from build123d import *

# Parameters (mm, degrees)
SKETCH1_R                   = 1.5
BOSS_EXTRUDE3_DEPTH         = 20
M10X1_0_TAPPED_HOLE2_REACH  = 97.384
M10X1_0_TAPPED_HOLE2_BORE_R = 4.5
M10X1_0_TAPPED_HOLE3_REACH  = 97.384
M10X1_0_TAPPED_HOLE3_BORE_R = 4.5
M10X1_0_TAPPED_HOLE4_REACH  = 97.514
M10X1_0_TAPPED_HOLE4_BORE_R = 4.5
M10X1_0_TAPPED_HOLE5_REACH  = 97.514
M10X1_0_TAPPED_HOLE5_BORE_R = 4.5


with BuildPart() as part:
    # Sketch1 → Boss-Extrude3 (new body)
    with BuildSketch(Plane(origin=(0, 0, 0), x_dir=(1, 0, 0), z_dir=(0, 1, 0))):
        with BuildLine():
            Line((-44.503051854, 39.975242963), (-45, 40))
            ThreePointArc((-45, 40), (-48.535533906, 38.535533906), (-50, 35))
            Line((-50, 35), (-49.953621428, 34.32056292))
            Line((-49.953621428, 34.32056292), (-47.610889869, 0))
            Line((-47.610889869, 0), (-49.953621428, -34.32056292))
            Line((-49.953621428, -34.32056292), (-50, -35))
            ThreePointArc((-50, -35), (-48.535533906, -38.535533906), (-45, -40))
            Line((-45, -40), (0, -37.473505635))
            Line((0, -37.473505635), (45, -40))
            ThreePointArc((45, -40), (48.535533906, -38.535533906), (50, -35))
            Line((50, -35), (49.982372149, -34.580514872))
            Line((49.982372149, -34.580514872), (48.529209365, 0))
            Line((48.529209365, 0), (49.982372149, 34.580514872))
            Line((49.982372149, 34.580514872), (50, 35))
            ThreePointArc((50, 35), (48.535533906, 38.535533906), (45, 40))
            Line((45, 40), (44.503051854, 39.975242963))
            Line((44.503051854, 39.975242963), (0, 37.758183271))
            Line((0, 37.758183271), (-44.503051854, 39.975242963))
        make_face()
        with Locations(Location((-45, -35, 0), (0, 0, 270))):
            Circle(SKETCH1_R, mode=Mode.SUBTRACT)
        with Locations(Location((45, -35, 0), (0, 0, 270))):
            Circle(SKETCH1_R, mode=Mode.SUBTRACT)
        with Locations(Location((-45, 35, 0), (0, 0, 270))):
            Circle(SKETCH1_R, mode=Mode.SUBTRACT)
        with BuildLine():
            Line((40.685277967, -32.473505635), (-40.685277967, -32.473505635))
            ThreePointArc((-40.685277967, -32.473505635), (-41.520684905, -31.409127338), (-42.610889869, -30.607716678))
            Line((-42.610889869, -30.607716678), (-42.610889869, 30.607716678))
            ThreePointArc((-42.610889869, 30.607716678), (-41.406196107, 31.523712673), (-40.530743043, 32.758183271))
            Line((-40.530743043, 32.758183271), (40.530743043, 32.758183271))
            ThreePointArc((40.530743043, 32.758183271), (41.770434724, 31.182945097), (43.529209365, 30.221216169))
            Line((43.529209365, 30.221216169), (43.529209365, -30.221216169))
            ThreePointArc((43.529209365, -30.221216169), (41.895770439, -31.080336898), (40.685277967, -32.473505635))
        make_face(mode=Mode.SUBTRACT)
        with Locations(Location((45, 35, 0), (0, 0, 270))):
            Circle(SKETCH1_R, mode=Mode.SUBTRACT)
    extrude(amount=BOSS_EXTRUDE3_DEPTH)

    # M10x1.0 Tapped Hole2 bore → M10x1.0 Tapped Hole2 (cut, up to next)
    with BuildSketch(Plane(origin=(2.097313344, 0, 37.355753405), x_dir=(0.9984276240489233, 0, -0.05605603924665131), z_dir=(0.05605603924665131, 0, 0.9984276240489233)), mode=Mode.PRIVATE) as m10x1_0_tapped_hole2_sk1:
        with Locations((-24.636050477, 10)):
            Circle(M10X1_0_TAPPED_HOLE2_BORE_R)
    m10x1_0_tapped_hole2_tool1 = extrude(m10x1_0_tapped_hole2_sk1.sketch, amount=-M10X1_0_TAPPED_HOLE2_REACH, mode=Mode.PRIVATE) & part.part
    add(m10x1_0_tapped_hole2_tool1.solids().sort_by_distance((-22.5, 10, 38.736753))[0], mode=Mode.SUBTRACT)

    # M10x1.0 Tapped Hole3 bore → M10x1.0 Tapped Hole3 (cut, up to next)
    with BuildSketch(Plane(origin=(-2.097313344, 0, 37.355753405), x_dir=(0.9984276240489233, 0, 0.056056039246651354), z_dir=(-0.056056039246651354, 0, 0.9984276240489233)), mode=Mode.PRIVATE) as m10x1_0_tapped_hole3_sk1:
        with Locations((24.636050477, 10)):
            Circle(M10X1_0_TAPPED_HOLE3_BORE_R)
    m10x1_0_tapped_hole3_tool1 = extrude(m10x1_0_tapped_hole3_sk1.sketch, amount=-M10X1_0_TAPPED_HOLE3_REACH, mode=Mode.PRIVATE) & part.part
    add(m10x1_0_tapped_hole3_tool1.solids().sort_by_distance((22.5, 10, 38.736753))[0], mode=Mode.SUBTRACT)

    # M10x1.0 Tapped Hole4 bore → M10x1.0 Tapped Hole4 (cut, up to next)
    with BuildSketch(Plane(origin=(-1.876385916, 0, -37.664705196), x_dir=(-0.9987613810598752, 0, 0.049756443837666), z_dir=(-0.049756443837666, 0, -0.9987613810598752)), mode=Mode.PRIVATE) as m10x1_0_tapped_hole4_sk1:
        with Locations((-24.406616413, 10)):
            Circle(M10X1_0_TAPPED_HOLE4_BORE_R)
    m10x1_0_tapped_hole4_tool1 = extrude(m10x1_0_tapped_hole4_sk1.sketch, amount=-M10X1_0_TAPPED_HOLE4_REACH, mode=Mode.PRIVATE) & part.part
    add(m10x1_0_tapped_hole4_tool1.solids().sort_by_distance((22.5, 10, -38.879092))[0], mode=Mode.SUBTRACT)

    # M10x1.0 Tapped Hole5 bore → M10x1.0 Tapped Hole5 (cut, up to next)
    with BuildSketch(Plane(origin=(1.876385916, 0, -37.664705196), x_dir=(-0.9987613810598767, 0, -0.04975644383763697), z_dir=(0.049756443837636964, 0, -0.9987613810598766)), mode=Mode.PRIVATE) as m10x1_0_tapped_hole5_sk1:
        with Locations((24.406616413, 10)):
            Circle(M10X1_0_TAPPED_HOLE5_BORE_R)
    m10x1_0_tapped_hole5_tool1 = extrude(m10x1_0_tapped_hole5_sk1.sketch, amount=-M10X1_0_TAPPED_HOLE5_REACH, mode=Mode.PRIVATE) & part.part
    add(m10x1_0_tapped_hole5_tool1.solids().sort_by_distance((-22.5, 10, -38.879092))[0], mode=Mode.SUBTRACT)


solid = part.part
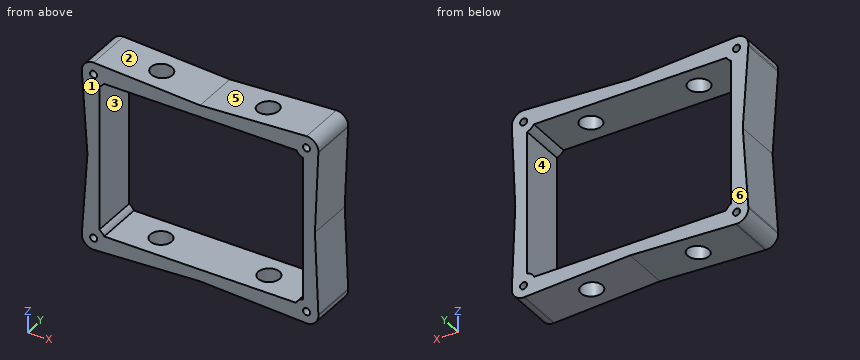
Design review of the part built by this model. Coordinates are the model's own, in mm. Face numbers are marked on the shaded views. A direction names the side the tool comes from. Round coordinates to 2 decimals unless told otherwise and drop trailing zeros. Order: outer loops, then holes, each group sorted by start corner. A loop starts at its lowest first (then second) coordinate and runs counter-clockwise, first axis right, second up.
1) Consider section C-C (x = 15.5). State the section outline as (y, z) points, plus the area to 3 significant figures.
The answers:
outline: (0, -38.53) - (20, -38.53) - (20, -32.76) - (0, -32.76) - close; (0, 32.47) - (20, 32.47) - (20, 38.34) - (0, 38.34) - close
area: 233 mm2
2) For L1, parallel to X at y = 2.75, z = -35; L2, parallel to X at y = 8, z = -35; L3, parallel to Z at x = -16, y = 13.75, list the stretches that pass through material, from the lowest coordinate up.
The answers:
L1: x = -50 to -46.5, -43.5 to 43.5, 46.5 to 50
L2: x = -50 to -46.5, -43.5 to -26.73, -18.66 to 18.66, 26.73 to 43.5, 46.5 to 50
L3: z = -38.56 to -32.76, 32.47 to 38.37
3) Consider section B-B (z = -3). State the section outline as (x, y) points, plus the area to 3 significant figures.
The answers:
outline: (-47.82, 0) - (-42.61, 0) - (-42.61, 20) - (-47.82, 20) - close; (43.53, 0) - (48.66, 0) - (48.66, 20) - (43.53, 20) - close
area: 207 mm2
4) Draft analysis for pull direction Z (two halves, no side actions). For the marked faces 4, 5 and 6, state which applies: released by +Z, released by -Z, zero draft, split by the parting line, or undercut.
The answers:
face 4: undercut
face 5: released by +Z
face 6: zero draft
5) Consider section A-A (y = 16.75). State the section outline as (x, z) points.
The answers:
outline: (-50, -35) arc R5 ccw to (-45, -40) - (0, -37.76) - (45, -40) arc R5 ccw to (50, -35) - (48.53, 0) - (50, 35) arc R5 ccw to (45, 40) - (0, 37.47) - (-45, 40) arc R5 ccw to (-50, 35) - (-47.61, 0) - close; hole circle Ø3 at (-45, -35); hole circle Ø3 at (-45, 35); hole (-42.61, -30.61) arc R5 cw to (-40.53, -32.76) - (40.53, -32.76) arc R5 cw to (43.53, -30.22) - (43.53, 30.22) arc R5 cw to (40.69, 32.47) - (-40.69, 32.47) arc R5 cw to (-42.61, 30.61) - close; hole circle Ø3 at (45, -35); hole circle Ø3 at (45, 35)
6) Machinability: for the marked faces 1, 2 and 3, which of the approach directions +Z, -Z, +X, -X, +Y, -Y give a long, thin tool a straight path to every point of the face, cutting with its end or side? Answer none if there is none.
The answers:
face 1: +Z, -Z, +X, -X, -Y
face 2: +Z, +Y, -Y
face 3: +Y, -Y
7) Clearance check with flat-ended pins moving along their axes: pin 1 Ø1.8 at (x, z) = (-45, -35) entering from +Y; pin 2 Ø1 at (x, y) = (-8.5, 16.5) entering from +Z; pin 3 Ø6 at (x, y) = (-15.5, 8.5) entering from +Z; pin 4 Ø3 at (x, y) = (14, 6) entering from -Z. State where each tip first meets the part, or that it passes through.
The answers:
pin 1: passes through
pin 2: stops at z = 37.98
pin 3: stops at z = 38.51
pin 4: stops at z = -38.53
8) Consider section D-D (y = 11.75). Count the separate pieces of the cut face and the enclosed holes in it, plus the area to 3 significant figures.
The answers:
separate pieces: 4
enclosed holes: 4
area: 1,790 mm2
